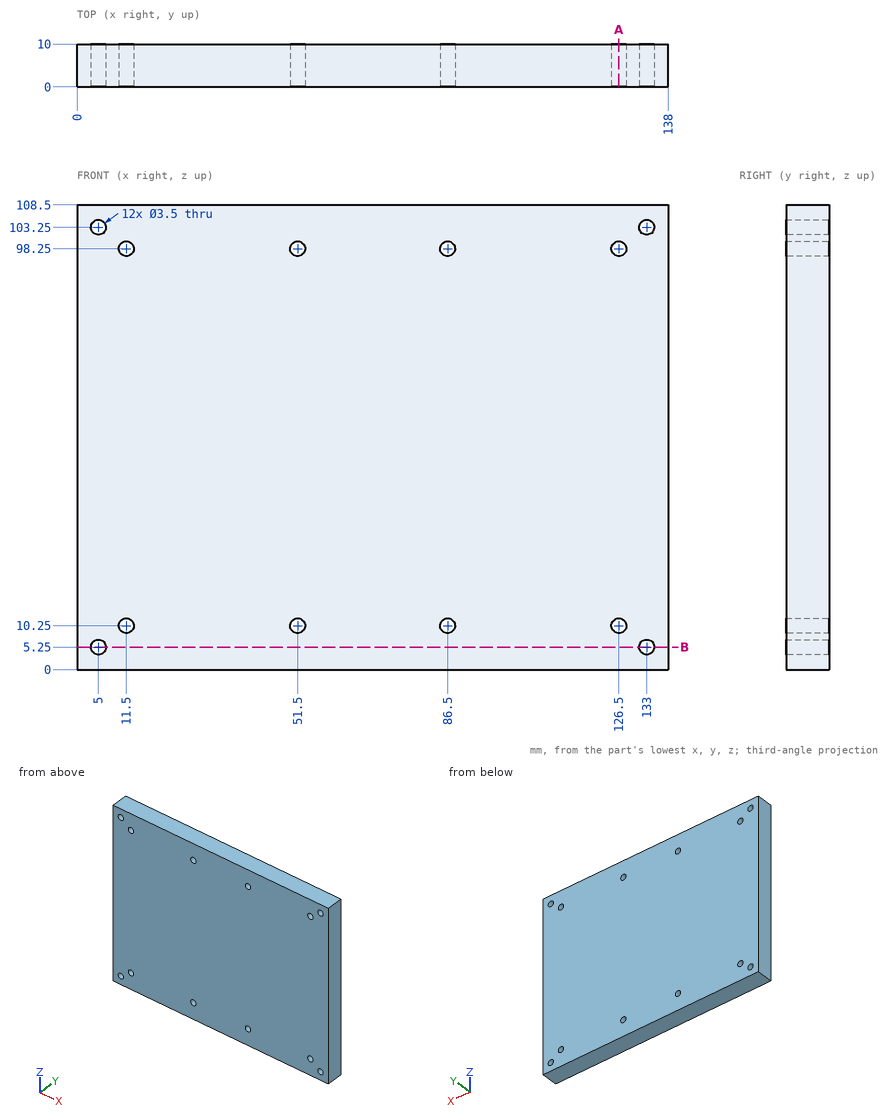
The figure shows three views and two pictorial views of one solid part (mm, origin at its lowest corner). Answer the questions. Coordinates: 2 decimals unless noted, no trailing zeros. Write each loop counter-clockwise with the first axis right and the second up, starting at its lowest first coordinate (ties: lowest second). Pieces come first, ordered by that corner, then holes. Notation, with made-up numbers: (59, 63) -> (91, 63) arc R35 cw to (91, 99) -> close; hole circle Ø1 at (47.5, 41.5). An arc over 180 degrees is marked (long way). Return JSON: item names as keys, results as strings.
1. Find the intervals of material crossed by line 1 along X through (y, z) = (2.75, 103.25); line 2 along X through (y, z) = (2.75, 10.25); line 3 along Z through (x, y) = (5, 6.5), in increasing order. Write a range as from..to.
Found:
{"line 1": "0..3.25, 6.75..131.25, 134.75..138", "line 2": "0..9.75, 13.25..49.75, 53.25..84.75, 88.25..124.75, 128.25..138", "line 3": "0..3.5, 7..101.5, 105..108.5"}
2. This flat-tipped pin is pushed along its axis until it touches: P1, Ø3, axis at x = 51.5, z = 10.25, coming from the +Y side. Where does it stop, or does it pass through?
Found:
{"P1": "through"}
3. A cutting plane is placed at A-A (x = 126.5). Determine the outline of the cut face in (y, z).
Found:
{"outline": "(0, 0) -> (10, 0) -> (10, 8.5) -> (0, 8.5) -> close; (0, 12) -> (10, 12) -> (10, 96.5) -> (0, 96.5) -> close; (0, 100) -> (10, 100) -> (10, 108.5) -> (0, 108.5) -> close"}
4. A cutting plane is placed at B-B (z = 5.25). Determine the outline of the cut face in (x, y), and give its area (3 significant figures).
Found:
{"outline": "(0, 0) -> (3.25, 0) -> (3.25, 10) -> (0, 10) -> close; (6.75, 0) -> (131.25, 0) -> (131.25, 10) -> (6.75, 10) -> close; (134.75, 0) -> (138, 0) -> (138, 10) -> (134.75, 10) -> close", "area": "1,310 mm2"}
